For this review, take the finished solid that the model builds, in its own axes (mm). Face numbers are marked on the shaded views. A direction names the side the tool comes from. Give positions to 0.01 mm unless a question says otherwise; leave off trailing zeros. Loops run counter-clockwise (first coordinate to the right, second up) from the corner with the lowest first, then second, coordinate; pieces in that order, holes last. Notation, with made-up numbers: (-32.5, -28.5) -> (-7.5, -28.5) arc R27 ccw to (-7.5, 0.5) -> close; hole circle Ø10 at (66, -11.75). An arc over 180 degrees is marked (long way). One line per question, with ' | ' between items. Start each with the question number.
(1) Tool access review of the marked faces 5, 6 and 7: name each direction out of +Z, -Z, +X, -X, +Y, -Y from which nothing blocks a thin tool from reaching the whole face with its end or side.
(2) Wall thickness on probe 1 along Y at (x, z) = (0, -0.6); probe 2 along Z at (x, y) = (2.25, 7.25); probe 3 along X at (y, z) = (9.25, -6): over which ranges is each line inside the solid? List them lowest first.
(3) Consider section A-A (x = 6.75). Write out the cut boundary in (y, z).
(4) Consider section B-B (y = 9.48). Write out the cut boundary in (x, z).
(5) Draft analysis for pull direction Y (two halves, no side actions). For the marked faces 1, 2, 3 and 4, state which applies: +Y half, -Y half, draft (parallel to the pull), parting line (faces both ways), or undercut.
(6) Insertion check: P1, Ø3.5, axis at y = 7, z = -10.5, coming from the -X side; P2, Ø1.2, axis at x = 5.5, z = -10, coming from the -Y side; P3, Ø3, axis at x = 5.5, y = 13, coming from the -Z side; P4, Ø1.6, axis at x = 0, y = 9.48, coming from the -Z side. Each pin has a flat end and moves straight along its axis. Give the tip position at first contact, or say it passes through.
(7) Consider section C-C (z = -4.5). Write out the cut boundary in (x, y), and give its area (3 significant figures).
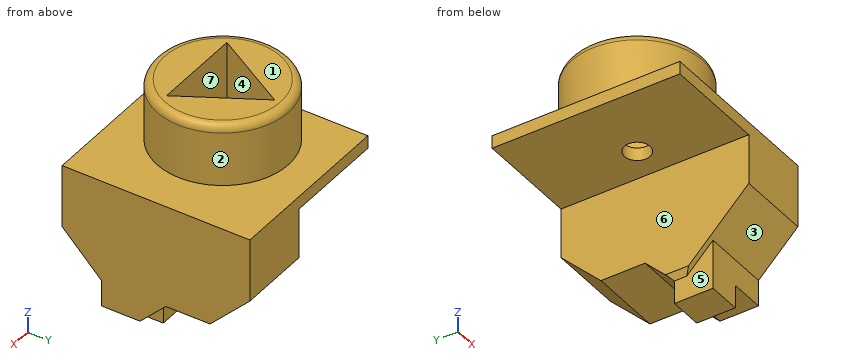
from build123d import *

# Parameters (mm, degrees)
SKETCH_2_R          = 5.1
EXTRUDE_1_DEPTH     = 4.8
SKETCH_3_W          = 11
SKETCH_3_H          = 14.6
EXTRUDE_2_DEPTH     = 1
SKETCH_4_R          = 1.5
EXTRUDE_3_DEPTH     = 10.8
CUT_EXTRUDE_1_DEPTH = 10.8
FILLET_1_R          = 0.6
CUT_EXTRUDE_2_DEPTH = 4.8
SKETCH_7_R          = 1
CUT_EXTRUDE_3_DEPTH = 1
SKETCH_8_W          = 3
SKETCH_8_H          = 14.6
EXTRUDE_4_DEPTH     = 7
CHAMFER_1_SIZE      = 3.1
SKETCH_9_W          = 2.584868303
SKETCH_9_H          = 3
EXTRUDE_5_DEPTH     = 10
CHAMFER_3_SIZE      = 2
CHAMFER_4_SIZE      = 2
EXTRUDE_6_DEPTH     = 2.7


with BuildPart() as part:
    # Эскиз2 → Бобышка-Вытянуть1 (new body)
    with BuildSketch(Plane.XY):
        with Locations((0, 9.48)):
            Circle(SKETCH_2_R)
    extrude(amount=EXTRUDE_1_DEPTH)

    # Эскиз3 → Бобышка-Вытянуть2 (add)
    with BuildSketch(Plane(origin=(0, 0, 0), x_dir=(-1, 0, 0), z_dir=(0, 0, -1))):
        with Locations((0, 9.78)):
            Rectangle(SKETCH_3_W, SKETCH_3_H)
    extrude(amount=EXTRUDE_2_DEPTH)

    # Эскиз4 → Бобышка-Вытянуть3 (add)
    with BuildSketch(Plane(origin=(0, 0, -1), x_dir=(-1, 0, 0), z_dir=(0, 0, -1))):
        with Locations(Location((-4.415131697, 7.038465404, 0), (0, 0, 223.676907922))):
            Circle(SKETCH_4_R)
    extrude(amount=EXTRUDE_3_DEPTH)

    # Эскиз5 → Вырез-Вытянуть1 (cut)
    with BuildSketch(Plane.XY.offset(-1)):
        with BuildLine():
            Line((5.5, 8.074351868), (5.5, 6.002578941))
            ThreePointArc((5.5, 6.002578941), (5.915131697, 7.038465404), (5.5, 8.074351868))
        make_face()
    extrude(amount=-CUT_EXTRUDE_1_DEPTH, mode=Mode.SUBTRACT)

    # Скругление1
    fillet_1_edges = [part.edges().sort_by_distance(p)[0] for p in [
        (-5.1, 9.48, 4.8),
    ]]
    fillet(fillet_1_edges, radius=FILLET_1_R)

    # Эскиз6 → Вырез-Вытянуть2 (cut)
    with BuildSketch(Plane.XY.offset(4.8)):
        Polygon((0.035898385, 13.542177826), (-3.464101615, 7.48), (3.535898385, 7.48), align=None)
    extrude(amount=-CUT_EXTRUDE_2_DEPTH, mode=Mode.SUBTRACT)

    # Эскиз7 → Вырез-Вытянуть3 (cut)
    with BuildSketch(Plane.XY):
        with Locations((0, 9.48)):
            Circle(SKETCH_7_R)
    extrude(amount=-CUT_EXTRUDE_3_DEPTH, mode=Mode.SUBTRACT)

    # Эскиз8 → Бобышка-Вытянуть4 (add)
    with BuildSketch(Plane(origin=(0, 0, -1), x_dir=(-1, 0, 0), z_dir=(0, 0, -1))):
        with Locations((-4, 9.78)):
            Rectangle(SKETCH_8_W, SKETCH_8_H)
    extrude(amount=EXTRUDE_4_DEPTH)

    # Фаска1
    # the kernel refuses this chamfer: 3.1 mm, written as the material it takes off along each edge
    with BuildSketch(Plane(origin=(-5.472217263, 2.48, -8), x_dir=(0, -0.027495876610586382, 0.9996219169112966), z_dir=(1, 0, 0))) as chamfer_1_piece_1_section:
        Polygon((CHAMFER_1_SIZE * 0.999621916911, -CHAMFER_1_SIZE * 0.0274958766106), (-CHAMFER_1_SIZE * 0.0274958766106, -CHAMFER_1_SIZE * 0.999621916911), (0, 0), align=None)
    chamfer_1_piece_1 = extrude(amount=18.944434525, mode=Mode.PRIVATE)
    chamfer_1_piece_1 = chamfer_1_piece_1 - Plane(origin=(4.415131697, 7.038465404, -6.977511347), x_dir=(0.7232455354515278, -0.6905909755053515, 0), z_dir=(0, 0, 1)) * Cylinder(1.5, 51, mode=Mode.PRIVATE)
    add(chamfer_1_piece_1, mode=Mode.SUBTRACT)
    with BuildSketch(Plane(origin=(13.472217263, 17.08, -8), x_dir=(0, -0.9996219169112966, -0.027495876610586514), z_dir=(-1, 0, 0))) as chamfer_1_piece_2:
        Polygon((CHAMFER_1_SIZE * 0.999621916911, CHAMFER_1_SIZE * 0.0274958766106), (-CHAMFER_1_SIZE * 0.0274958766106, CHAMFER_1_SIZE * 0.999621916911), (0, 0), align=None)
    extrude(amount=18.944434525, mode=Mode.SUBTRACT)

    # Эскиз9 → Бобышка-Вытянуть5 (add)
    with BuildSketch(Plane(origin=(0, 0, -11.8), x_dir=(-1, 0, 0), z_dir=(0, 0, -1))):
        with Locations((-4.207565848, 7.038465404)):
            Rectangle(SKETCH_9_W, SKETCH_9_H)
    extrude(amount=-EXTRUDE_5_DEPTH)

    # Фаска3
    chamfer_3_edges = [part.edges().sort_by_distance(p)[0] for p in [
        (4.207565848, 8.538465404, -8),
    ]]
    chamfer(chamfer_3_edges, length=CHAMFER_3_SIZE)

    # Фаска4
    # the kernel refuses this chamfer: 2 mm, written as the material it adds along each edge
    with BuildSketch(Plane(origin=(2.915131697, 15.68183138, -8), x_dir=(-0.9996219169112968, 6.965053790802993e-15, 0.027495876610586487), z_dir=(0, -1, 0))) as chamfer_4_piece_1_section:
        Polygon((CHAMFER_4_SIZE * 0.999621916911, CHAMFER_4_SIZE * 0.0274958766106), (-CHAMFER_4_SIZE * 0.0274958766106, CHAMFER_4_SIZE * 0.999621916911), (0, 0), align=None)
    chamfer_4_piece_1 = extrude(amount=15.245197356, mode=Mode.PRIVATE)
    chamfer_4_piece_1 = split(chamfer_4_piece_1, bisect_by=Plane(origin=(2.5, 9.220354444, -8.636221921), z_dir=(1, 0, 0)), keep=Keep.TOP, mode=Mode.PRIVATE)
    chamfer_4_piece_1 = split(chamfer_4_piece_1, bisect_by=Plane(origin=(2.728922141, 9.561298963, -8.977166441), z_dir=(0, -0.7071067811865476, 0.7071067811865476)), keep=Keep.TOP, mode=Mode.PRIVATE)
    chamfer_4_piece_1 = split(chamfer_4_piece_1, bisect_by=Plane(origin=(2.728922141, 8.538465404, -8.636221921), z_dir=(0, 1, 0)), keep=Keep.TOP, mode=Mode.PRIVATE)
    add(chamfer_4_piece_1)
    with BuildSketch(Plane(origin=(2.915131697, 15.68183138, -8), x_dir=(-0.9996219169112968, 6.965053790802993e-15, 0.027495876610586487), z_dir=(0, -1, 0))) as chamfer_4_piece_2_section:
        Polygon((CHAMFER_4_SIZE * 0.999621916911, CHAMFER_4_SIZE * 0.0274958766106), (-CHAMFER_4_SIZE * 0.0274958766106, CHAMFER_4_SIZE * 0.999621916911), (0, 0), align=None)
    chamfer_4_piece_2 = extrude(amount=15.245197356, mode=Mode.PRIVATE)
    chamfer_4_piece_2 = split(chamfer_4_piece_2, bisect_by=Plane(origin=(2.5, 7.443880943, -8.769342974), z_dir=(1, 0, 0)), keep=Keep.TOP, mode=Mode.PRIVATE)
    chamfer_4_piece_2 = split(chamfer_4_piece_2, bisect_by=Plane(origin=(2.735166787, 6.896611958, -9.316611958), z_dir=(0, 0.7071067811862648, 0.7071067811868302)), keep=Keep.TOP, mode=Mode.PRIVATE)
    chamfer_4_piece_2 = split(chamfer_4_piece_2, bisect_by=Plane(origin=(2.735166787, 8.606501686, -9.931963718), z_dir=(0, -0.7071067811865476, 0.7071067811865476)), keep=Keep.TOP, mode=Mode.PRIVATE)
    chamfer_4_piece_2 = split(chamfer_4_piece_2, bisect_by=Plane(origin=(2.735166787, 8.538465404, -8.769342974), z_dir=(0, -1, 0)), keep=Keep.TOP, mode=Mode.PRIVATE)
    add(chamfer_4_piece_2)

    # Эскиз10 → Бобышка-Вытянуть6 (add)
    with BuildSketch(Plane(origin=(5.5, 0, 0), x_dir=(0, 0, -1), z_dir=(1, 0, 0))):
        Polygon((10, 5.538465404), (10, 8.538465404), (8, 10.538465404), (8, 13.98), (4.9, 17.08), (0, 17.08), (0, 2.48), (4.9, 2.48), (7.958465404, 5.538465404), align=None)
    extrude(amount=EXTRUDE_6_DEPTH)


solid = part.part
A:
1) face 5: -Z, -X, -Y | face 6: -Z, -X, +Y, -Y | face 7: +Z
2) probe 1: y = 2.48 to 8.48, 10.48 to 17.08 | probe 2: z = -1 to 4.8 | probe 3: x = 2.5 to 8.2
3) outline: (2.48, -4.9) -> (5.54, -7.96) -> (5.54, -10) -> (8.54, -10) -> (10.54, -8) -> (13.98, -8) -> (17.08, -4.9) -> (17.08, 0) -> (2.48, 0) -> close
4) outline: (-5.5, -1) -> (-1, -1) -> (-1, 0) -> (-2.31, 0) -> (-2.31, 4.8) -> (-4.5, 4.8) arc R0.6 ccw to (-5.1, 4.2) -> (-5.1, 0) -> (-5.5, 0) -> close; (1, -1) -> (2.5, -1) -> (2.5, -9.06) -> (8.2, -9.06) -> (8.2, 0) -> (5.1, 0) -> (5.1, 4.2) arc R0.6 ccw to (4.5, 4.8) -> (2.38, 4.8) -> (2.38, 0) -> (1, 0) -> close
5) face 1: draft | face 2: parting line | face 3: -Y half | face 4: undercut
6) P1: stops at x = 2.5 | P2: stops at y = 5.54 | P3: stops at z = -8 | P4: passes through
7) outline: (2.5, 2.48) -> (8.2, 2.48) -> (8.2, 17.08) -> (2.5, 17.08) -> close | area: 83.2 mm^2
